The drawing under review shows one solid part. Ordinate dimensions are in mm from its lowest x, y, z. Give positions to 0.01 mm unless a question says otherwise; leave off trailing zeros. Loops run counter-clockwise (first coordinate to the right, second up) from the corner with the lowest first, then second, coordinate; pieces in that order, holes last. Notation, with made-up numbers: (-6.5, 49) - (26.5, 49) arc R24 cw to (26.5, 80) - close; hole circle Ø5 at (28.25, 49). An arc over 180 degrees is marked (long way). One line per item, written item: value. Start each with the question number.
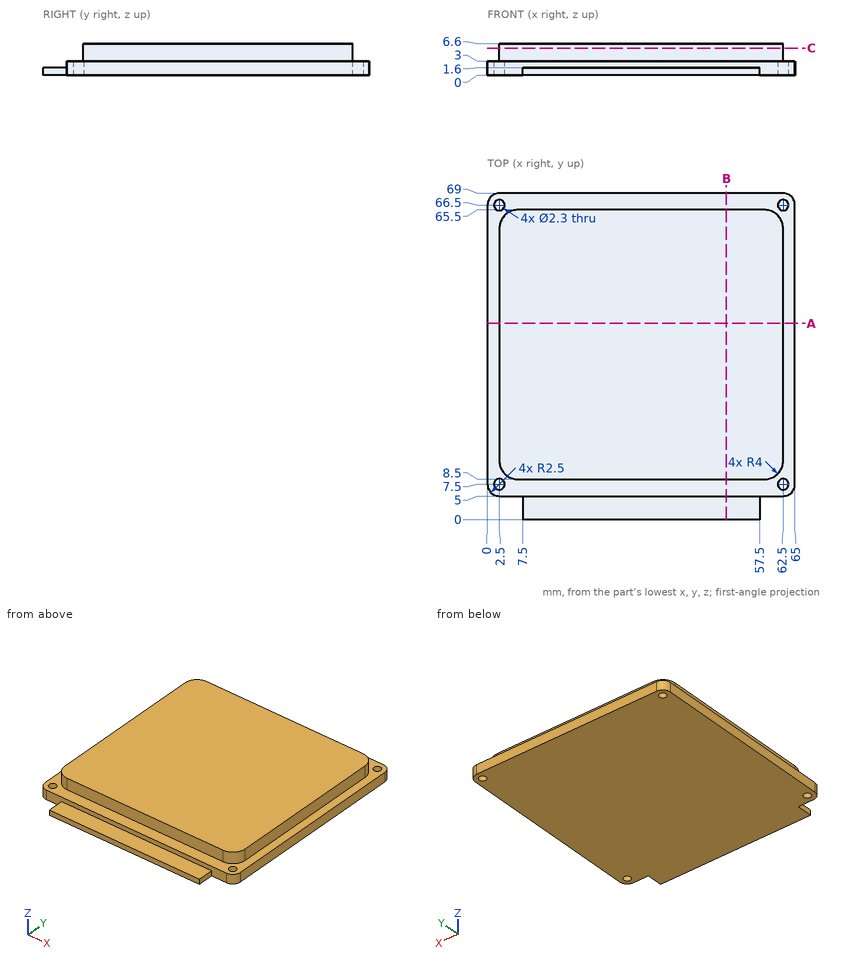
(1) Take a section at C-C on z = 5.75. State the section outline as (x, y) points.
(2) Take a section at A-A on y = 41.5. State the section outline as (x, z) points.
(3) For pin 1 Ø4 at (x, y) = (21, 54.5) entering from -Z; pin 2 Ø1 at (x, z) = (20.5, 4.5) entering from -Y; pin 3 Ø2.5 at (x, y) = (2.5, 7.5) entering from +Z; pin 4 Ø0.8 at (y, z) = (3.5, 1) entering from -X, all flat-tipped, find the tip position at first contact; note any pin that passes through.
(4) Take a section at B-B on x = 50.5. State the section outline as (y, z) points.
(5) To check wall thickness, follow L1, parallel to X at y = 66.5, z = 1; L2, parallel to Y at x = 34.5, z = 5.25; L3, parallel to Y at x = 45, z = 2. State the ranges of each line that lie inside material, in increasing order. Write a range as from..to.
Here are the results:
1. outline: (2.5, 12.5) arc R4 ccw to (6.5, 8.5) - (58.5, 8.5) arc R4 ccw to (62.5, 12.5) - (62.5, 61.5) arc R4 ccw to (58.5, 65.5) - (6.5, 65.5) arc R4 ccw to (2.5, 61.5) - close
2. outline: (0, 0) - (65, 0) - (65, 3) - (62.5, 3) - (62.5, 6.6) - (2.5, 6.6) - (2.5, 3) - (0, 3) - close
3. pin 1: z = 0
3. pin 2: y = 8.5
3. pin 3: z = 3
3. pin 4: x = 7.5
4. outline: (0, 0) - (69, 0) - (69, 3) - (65.5, 3) - (65.5, 6.6) - (8.5, 6.6) - (8.5, 3) - (5, 3) - (5, 1.6) - (0, 1.6) - close
5. L1: 0..1.35, 3.65..61.35, 63.65..65
5. L2: 8.5..65.5
5. L3: 5..69
